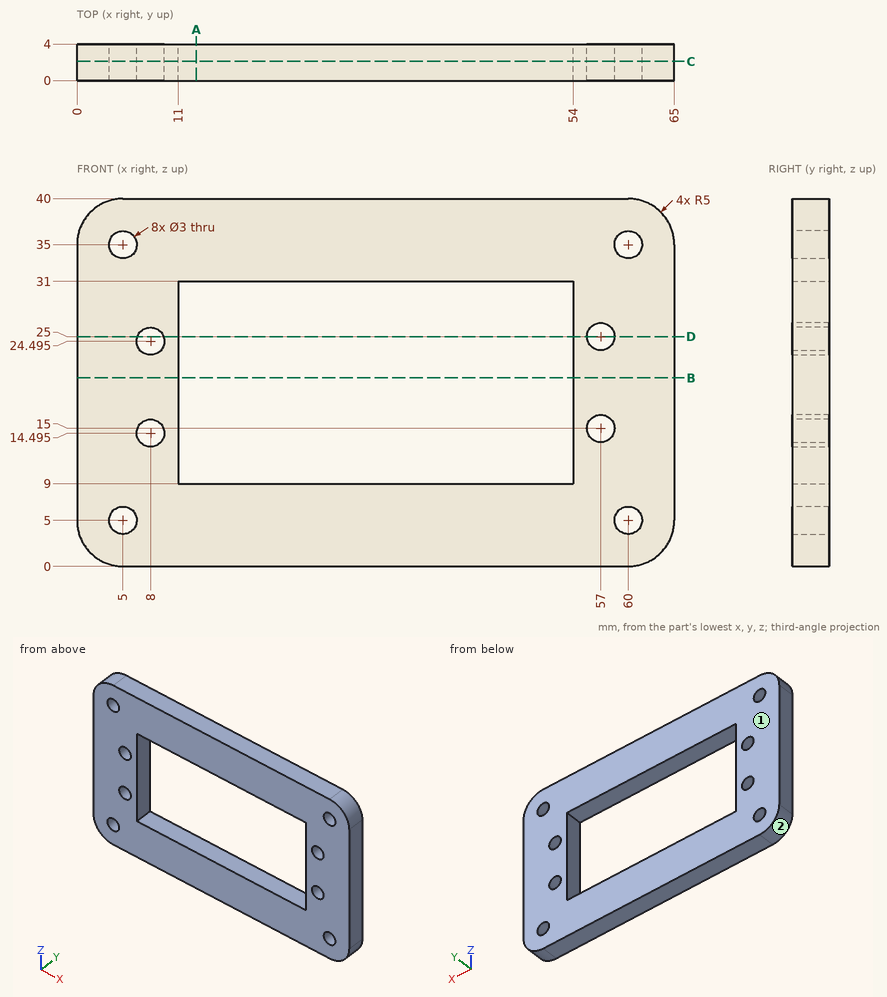
Here's the drawing with two shaded views (mm, measured from the low corner). I have some questions. Coordinates: 2 decimals unless noted, no trailing zeros. Order: outer loops, then holes, each group sorted by start corner. A loop starts at its lowest first (then second) coordinate and runs counter-clockwise, first axis right, second up. Notation, with made-up numbers: (-10.5, 29) - (37.5, 29) arc R25 ccw to (37.5, 55) - close; hole circle Ø1 at (31.5, 61). An arc over 180 degrees is marked (long way). Answer in a Markdown table with one row per item. Add a question column.
(1) If we section it at C-C, the plane y = 2.1: State how many separate pieces and enclosed holes the cut face has, then the cut area to 3 significant figures.
(2) If we section it at A-A, the plane x = 13: Please give me the cut outline in (y, z).
(3) If we section it at B-B, the plane z = 20.5: Please give me the cut outline in (x, y).
(4) If we mould it in two halves opening along Z, with no side actions, what happens to the marked faces 1 and 2? For each: released by +Z, released by -Z, zero draft, split by the parting line, or undercut.
(5) Will this pin go through, and if not, where does the flat tip stop? pin 1 (5 mm diameter, centred on x = 49, z = 26.5, fed in from -Y).
(6) I need wall thicknesses on L1, parallel to X at y = 1.05, z = 5; L2, parallel to Z at x = 47.5, y = 1.55; L3, parallel to X at y = 2.05, z = 27.5. Which ranges of each line are inside material? Lowest first, please.
(7) If we section it at D-D, the plane z = 25: Please give me the cut outline in (x, y).
Results are:
| question | item | result |
|---|---|---|
| 1 | separate pieces | 1 |
| 1 | enclosed holes | 9 |
| 1 | area | 1,580 mm2 |
| 2 | outline | (0, 0) - (4, 0) - (4, 9) - (0, 9) - close; (0, 31) - (4, 31) - (4, 40) - (0, 40) - close |
| 3 | outline | (0, 0) - (11, 0) - (11, 4) - (0, 4) - close; (54, 0) - (65, 0) - (65, 4) - (54, 4) - close |
| 4 | face 1 | zero draft |
| 4 | face 2 | released by -Z |
| 5 | pin 1 | passes through |
| 6 | L1 | x = 0 to 3.5, 6.5 to 58.5, 61.5 to 65 |
| 6 | L2 | z = 0 to 9, 31 to 40 |
| 6 | L3 | x = 0 to 11, 54 to 65 |
| 7 | outline | (0, 0) - (6.59, 0) - (6.59, 4) - (0, 4) - close; (9.41, 0) - (11, 0) - (11, 4) - (9.41, 4) - close; (54, 0) - (55.5, 0) - (55.5, 4) - (54, 4) - close; (58.5, 0) - (65, 0) - (65, 4) - (58.5, 4) - close |
